from build123d import *

# Parameters (mm, degrees)
ESQUISSE6_W        = 28.284271248
ESQUISSE6_H        = 28.284271248
BOSS_EXTRU_2_DEPTH = 25
BOSS_EXTRU_2_TAPER = 22.5
ESQUISSE7_R        = 2.8
BOSS_EXTRU_3_DEPTH = 3


with BuildPart() as part:
    # Esquisse6 → Boss.-Extru.2 (new body)
    with BuildSketch(Plane(origin=(0, 0, 0), x_dir=(1, 0, 0), z_dir=(0, 1, 0))):
        Rectangle(ESQUISSE6_W, ESQUISSE6_H)
    extrude(amount=BOSS_EXTRU_2_DEPTH, taper=BOSS_EXTRU_2_TAPER)

    # Congé3
    # a fillet whose section is not a circle: 15, 9 mm, written as the material it takes off along each edge
    with BuildSketch(Plane(origin=(-35.056698922, 25, 3.786796564), x_dir=(0, -0.9238795325112864, 0.38268343236509067), z_dir=(1, 0, 0)), Plane(origin=(-3.786796564, 25, -35.056698922), x_dir=(-0.3826834323650906, -0.9238795325112864, 0), z_dir=(0, 0, 1)), Plane(origin=(35.056698922, 25, -3.786796564), x_dir=(0, -0.9238795325112864, -0.38268343236509056), z_dir=(-1, 0, 0)), Plane(origin=(3.786796564, 25, 35.056698922), x_dir=(0.3826834323650906, -0.9238795325112864, 0), z_dir=(0, 0, -1))) as cong_3_piece_1:
        with BuildLine():
            Bezier((12.507960943, 0), (0, 0), (-1.350232045, 3.259748515), weights=[1, 1, 1])
            Line((-1.350232045, 3.259748515), (0, 0))
            Line((0, 0), (12.507960943, 0))
        make_face()
    extrude(amount=70.113397844, mode=Mode.SUBTRACT)

    # Esquisse7 → Boss.-Extru.3 (add)
    with BuildSketch(Plane.XZ):
        with Locations(Location((-10.606601718, 10.606601718, 0), (0, 0, 90))):
            Circle(ESQUISSE7_R)
        with Locations(Location((10.606601718, 10.606601718, 0), (0, 0, 90))):
            Circle(ESQUISSE7_R)
        with Locations(Location((10.606601718, -10.606601718, 0), (0, 0, 90))):
            Circle(ESQUISSE7_R)
        with Locations(Location((-10.606601718, -10.606601718, 0), (0, 0, 90))):
            Circle(ESQUISSE7_R)
    extrude(amount=BOSS_EXTRU_3_DEPTH)


solid = part.part
Input: part model. Units: mm. Frame: model coordinates. A direction names the side the tool comes from. Round coordinates to 2 decimals unless told otherwise and drop trailing zeros.
1) Reachability of faces 3 (the flat face through (-11, -3, 11)), 4 (the flat face through (0, 0, 0)) from +Z, -Z, +X, -X, +Y, -Y: full face, straight path, thin tool, end or side. Return the list, or none.
2) Contact query for flat-ended pins moving along their axis: P1, Ø2, axis at x = 2.5, z = 8.5, coming from the +Y side; P2, Ø4, axis at x = 4, y = 20, coming from the +Z side; P3, Ø6, axis at x = -6, y = 14.5, coming from the +Z side. Output: stop coordinate, or through.
3) Ray query, L1, parallel to Z at x = 1, y = 7; L2, parallel to Y at x = 12.25, z = 0.5; L3, parallel to X at y = 5.5, z = -3.75. Return the intervals inside material, ascending.
4) Draft query along X for faces 1 (the flat face through (-11, -3, -11)), 2 (the cylindrical face through (7.83, -1.48, -10.97)). Return one class per face: pulls with the +X half, pulls with the -X half, needs draft (parallel to the pull), parting line crosses it, or undercut.
Geometry says:
1. face 3: +Z, -Z, +X, -X, -Y
1. face 4: -Y
2. P1: stops at y = 15.93
2. P2: stops at z = 6.51
2. P3: stops at z = 9.38
3. L1: z = -11.24 to 11.24
3. L2: y = 0 to 4.57
3. L3: x = -11.86 to 11.86
4. face 1: needs draft
4. face 2: undercut
